from build123d import *

# Parameters (mm, degrees)
SKETCH1_R           = 0.95
SKETCH1_R_2         = 3.175
SKETCH1_RX          = 32.5
SKETCH1_RY          = 15.3
BOSS_EXTRUDE1_DEPTH = 6.35
SKETCH2_W           = 15.875
SKETCH2_H           = 159.01875
BOSS_EXTRUDE2_DEPTH = 3.175
SKETCH3_W           = 15.875
SKETCH3_H           = 6.35
BOSS_EXTRUDE3_DEPTH = 25.4
SKETCH4_R           = 3.175
CUT_EXTRUDE1_DEPTH  = 123.890515655
FILLET2_R           = 6.35


with BuildPart() as part:
    # Sketch1 → Boss-Extrude1 (new body)
    with BuildSketch(Plane.XY):
        Polygon((-50.8, -79.509375), (-50.8, 79.509375), (-34.925, 79.509375), (-34.925, 16.5), (34.925, 16.5), (34.925, 79.509375), (50.8, 79.509375), (50.8, -79.509375), (34.925, -79.509375), (34.925, -39.5), (-34.925, -39.5), (-34.925, -79.509375), align=None)
        with Locations((29, 13)):
            Circle(SKETCH1_R, mode=Mode.SUBTRACT)
        with Locations((29, -36)):
            Circle(SKETCH1_R, mode=Mode.SUBTRACT)
        with Locations((-29, -36)):
            Circle(SKETCH1_R, mode=Mode.SUBTRACT)
        with Locations((-29, 13)):
            Circle(SKETCH1_R, mode=Mode.SUBTRACT)
        with Locations((-42.8625, 71.571875)):
            Circle(SKETCH1_R_2, mode=Mode.SUBTRACT)
        with Locations(Location((42.8625, 71.571875, 0), (0, 0, 180))):
            Circle(SKETCH1_R_2, mode=Mode.SUBTRACT)
        with Locations(Location((-42.8625, -71.571875, 0), (0, 0, 180))):
            Circle(SKETCH1_R_2, mode=Mode.SUBTRACT)
        with Locations((42.8625, -71.571875)):
            Circle(SKETCH1_R_2, mode=Mode.SUBTRACT)
        with Locations(Location((0, -11.5), (0, 0, 0))):
            Ellipse(SKETCH1_RX, SKETCH1_RY, mode=Mode.SUBTRACT)
    extrude(amount=BOSS_EXTRUDE1_DEPTH)

    # Sketch2 → Boss-Extrude2 (add)
    # profile 1 of 2: a face of its own
    with BuildSketch(Plane.XY.offset(6.35)):
        with Locations((-42.8625, 0)):
            Rectangle(SKETCH2_W, SKETCH2_H)
        Polygon((-48.4875, 68.324279736), (-42.8625, 65.076684472), (-37.2375, 68.324279736), (-37.2375, 74.819470264), (-42.8625, 78.067065528), (-48.4875, 74.819470264), align=None, mode=Mode.SUBTRACT)
        Polygon((-37.2375, -68.324279736), (-42.8625, -65.076684472), (-48.4875, -68.324279736), (-48.4875, -74.819470264), (-42.8625, -78.067065528), (-37.2375, -74.819470264), align=None, mode=Mode.SUBTRACT)
    # profile 2 of 2: a face of its own
    with BuildSketch(Plane.XY.offset(6.35)):
        with Locations((42.8625, 0)):
            Rectangle(SKETCH2_W, SKETCH2_H)
        Polygon((37.2375, -74.819470264), (37.2375, -68.324279736), (42.8625, -65.076684472), (48.4875, -68.324279736), (48.4875, -74.819470264), (42.8625, -78.067065528), align=None, mode=Mode.SUBTRACT)
        Polygon((48.4875, 74.819470264), (48.4875, 68.324279736), (42.8625, 65.076684472), (37.2375, 68.324279736), (37.2375, 74.819470264), (42.8625, 78.067065528), align=None, mode=Mode.SUBTRACT)
    extrude(amount=BOSS_EXTRUDE2_DEPTH)

    # Sketch3 → Boss-Extrude3 (add)
    with BuildSketch(Plane.XY.offset(9.525)):
        with Locations((-42.8625, -23.625)):
            Rectangle(SKETCH3_W, SKETCH3_H)
        with Locations((42.8625, -23.625)):
            Rectangle(SKETCH3_W, SKETCH3_H)
    extrude(amount=BOSS_EXTRUDE3_DEPTH)

    # Sketch4 → Cut-Extrude1 (cut, through all)
    with BuildSketch(Plane(origin=(0, -26.8, 0), x_dir=(1, 0, 0), z_dir=(0, 1, 0))):
        with Locations((-42.8625, -22.225)):
            Circle(SKETCH4_R)
        with Locations((42.8625, -22.225)):
            Circle(SKETCH4_R)
    extrude(amount=CUT_EXTRUDE1_DEPTH, mode=Mode.SUBTRACT)

    # Fillet2
    fillet2_edges = [part.edges().sort_by_distance(p)[0] for p in [
        (-50.8, -79.509375, 4.7625),
        (-50.8, 79.509375, 4.7625),
        (-34.925, 79.509375, 4.7625),
        (-34.925, 16.5, 3.175),
        (34.925, 16.5, 3.175),
        (34.925, 79.509375, 4.7625),
        (50.8, 79.509375, 4.7625),
        (50.8, -79.509375, 4.7625),
        (34.925, -79.509375, 4.7625),
        (34.925, -39.5, 3.175),
        (-34.925, -39.5, 3.175),
        (-34.925, -79.509375, 4.7625),
    ]]
    fillet(fillet2_edges, radius=FILLET2_R)


solid = part.part
Read the model definition and answer for the solid it produces. Units are mm, in the model's axes. A direction names the side the tool comes from. Round coordinates to 2 decimals unless told otherwise and drop trailing zeros. Order: outer loops, then holes, each group sorted by start corner. A loop starts at its lowest first (then second) coordinate and runs counter-clockwise, first axis right, second up. Notation, with made-up numbers: (85.25, 56) - (126.25, 56) arc R27 cw to (126.25, 91) - close; hole circle Ø3 at (11.5, -26). An arc over 180 degrees is marked (long way). Use one line per item in the form item = value. Start each with the question number.
(1) Flat-ended cylindrical pins translate along their axes: pin 1 Ø3 at (x, y) = (-29, -36) entering from +Z; pin 2 Ø17.5 at (x, y) = (-40, -40.5) entering from +Z (3 decimals); pin 3 Ø7 at (x, z) = (4.5, 3.5) entering from +Y; pin 4 Ø12 at (x, z) = (-27, 24.5) entering from -Y. Find the tip coordinate at first contact, or state that the pin passes through.
(2) The part is cut by section B-B (y = 39.5). Give the vertices of the cut face in (x, z) (3 decimals).
(3) Find the intervals of material crossed by line 1 along X through (y, z) = (-36, 3.75); line 2 along Y through (x, z) = (43, 6); line 3 along Y through (x, z) = (29, 4.75), in increasing order. Write a range as from..to.
(4) Determine the mould class of faces 6 (the face through (-50.8, 0, 7)), 7 (the face through (43.55, 74.67, 3.13)), 8 (the face through (-43, 30, 9.525)), 9 (the face through (48.89, -77.7, 4.83)) for opening direction X: +X half, -X half, draft (parallel to the pull), parting line (faces both ways), or undercut.
(5) The part is cut by section C-C (z = 3). Count the separate pieces of the cut face and the enclosed holes in it, then the cut area to 3 significant figures.
(6) For faces 1 (the face through (-43, -79.509, 5)), 2 (the face through (0, 16.5, 3)), 3 (the face through (-37.238, -72, 8)), 4 (the face through (0, 4, 6.35)), 5 (the face through (36.736, -77.6, 4.829)), determine the directions among +Z, -Z, +X, -X, +Y, -Y from which every point of the face is accessible in a straight line to the end or side of a thin tool.
(7) The part is cut by section A-A (z = 27). Give the vertices of the cut face in (x, y) (3 decimals), then the cut area to 3 significant figures.
Checked values:
q1.pin_1 = 6.35
q1.pin_2 = 9.525
q1.pin_3 = 16.5
q1.pin_4 = through
q2.outline = (-50.8, 0) - (-34.925, 0) - (-34.925, 9.525) - (-50.8, 9.525) - close; (34.925, 0) - (50.8, 0) - (50.8, 9.525) - (34.925, 9.525) - close
q3.line_1 = -50.8..-29.95, -28.05..28.05, 29.95..50.8
q3.line_2 = -79.51..-74.74, -68.4..68.4, 74.74..79.51
q3.line_3 = -39.51..-36.95, -35.05..-18.41, -4.59..12.05, 13.95..16.51
q4.face_6 = -X half
q4.face_7 = undercut
q4.face_8 = draft
q4.face_9 = +X half
q5.separate_pieces = 1
q5.enclosed_holes = 9
q5.area = 7,230 mm^2
q6.face_1 = +Z, -Z, +X, -X, -Y
q6.face_2 = +Z, -Z, +Y
q6.face_3 = +Z
q6.face_4 = +Z, +Y, -Y
q6.face_5 = +Z, -Z, -Y
q7.outline = (-50.8, -26.8) - (-34.925, -26.8) - (-34.925, -20.45) - (-50.8, -20.45) - close; (34.925, -26.8) - (50.8, -26.8) - (50.8, -20.45) - (34.925, -20.45) - close
q7.area = 202 mm^2
